Geometry: final body of the model. Coordinates: model frame, mm. A direction names the side the tool comes from. Give positions to 0.01 mm unless a question says otherwise; leave off trailing zeros. Order: outer loops, then holes, each group sorted by start corner. A loop starts at its lowest first (then second) coordinate and runs counter-clockwise, first axis right, second up. Notation, with made-up numbers: M -37.75,46.5 L -18.75,46.5 A22 cw -18.75,65.5 Z; hole C 48,59 d1. An arc over 180 degrees is marked long. Use CSV: the item, a comma, the result in double quotes.
```python
from build123d import *

# Parameters (mm, degrees)
SKETCH_2_R          = 1.65
SKETCH_2_R_2        = 6.3
EXTRUDE_1_DEPTH     = 5
SKETCH_4_W          = 4
SKETCH_4_H          = 55
EXTRUDE_3_DEPTH     = 54
CUT_EXTRUDE_1_DEPTH = 54


with BuildPart() as part:
    # 草图2 → 凸台-拉伸1 (new body)
    with BuildSketch(Plane.XY):
        Polygon((15.6, 35), (0, 35), (-15.6, 35), (-15.6, -20), (18.6, -20), (18.6, 35), align=None)
        with Locations((-9, -5)):
            Circle(SKETCH_2_R, mode=Mode.SUBTRACT)
        with Locations((0, -5)):
            Circle(SKETCH_2_R_2, mode=Mode.SUBTRACT)
        with Locations((9, -5)):
            Circle(SKETCH_2_R, mode=Mode.SUBTRACT)
    extrude(amount=EXTRUDE_1_DEPTH)

    # 草图4 → 凸台-拉伸3 (add)
    with BuildSketch(Plane.XY.offset(5)):
        with Locations((16.6, 7.5)):
            Rectangle(SKETCH_4_W, SKETCH_4_H)
    extrude(amount=EXTRUDE_3_DEPTH)

    # 草图6 → 切除-拉伸1 (cut)
    with BuildSketch(Plane(origin=(0, 0, 0), x_dir=(0, 0, -1), z_dir=(1, 0, 0))):
        Polygon((-59, 7.5), (-59, -20), (-5, -20), align=None)
        with BuildLine():
            ThreePointArc((-32.65, 20), (-31, 18.35), (-29.35, 20))
            Line((-29.35, 20), (-32.65, 20))
        make_face()
        with BuildLine():
            Line((-32.65, 20), (-29.35, 20))
            ThreePointArc((-29.35, 20), (-31, 21.65), (-32.65, 20))
        make_face()
        with BuildLine():
            ThreePointArc((-33.7, 20), (-40, 26.3), (-46.3, 20))
            Line((-46.3, 20), (-33.7, 20))
        make_face()
        with BuildLine():
            Line((-33.7, 20), (-46.3, 20))
            ThreePointArc((-46.3, 20), (-40, 13.7), (-33.7, 20))
        make_face()
        with BuildLine():
            ThreePointArc((-47.35, 20), (-49, 21.65), (-50.65, 20))
            Line((-50.65, 20), (-47.35, 20))
        make_face()
        with BuildLine():
            Line((-47.35, 20), (-50.65, 20))
            ThreePointArc((-50.65, 20), (-49, 18.35), (-47.35, 20))
        make_face()
    extrude(amount=CUT_EXTRUDE_1_DEPTH, mode=Mode.SUBTRACT)


solid = part.part
```
1. Pull-direction query (Z, two-part tool) for faces 1 (the face through (1, 8, 0)), 2 (the face through (16.572, 18.885, 47.784)), 3 (the face through (14.6, 13, 26)), 4 (the face through (16.572, 13.754, 39.18)); classes: +Z half, -Z half, draft (parallel to the pull), parting line (faces both ways), or undercut.
Answer:
face 1,"-Z half"
face 2,"undercut"
face 3,"draft"
face 4,"undercut"
2. Section D-D, the plane x = 11.5. Return the cut outline in (y, z), plus the area to 3 significant figures.
Answer:
outline,"M -20,0 L 35,0 L 35,5 L -20,5 Z"
area,"275 mm2"
3. Line query: line 1 (Y direction, x = -9, z = 2.15); line 2 (Y direction, x = 0, z = 3.8); line 3 (X direction, y = 11, z = 14.5). Output: solid intervals per line, ascending.
Answer:
line 1,"-20 to -6.65, -3.35 to 35"
line 2,"-20 to -11.3, 1.3 to 35"
line 3,"14.6 to 18.6"
4. Section B-B, the plane z = 43. Return the cut outline in (x, y), plus the area to 3 significant figures.
Answer:
outline,"M 14.6,-0.65 L 18.6,-0.65 L 18.6,14.46 L 14.6,14.46 Z; M 14.6,25.54 L 18.6,25.54 L 18.6,35 L 14.6,35 Z"
area,"98.3 mm2"
5. Section A-A, the plane x = 0. Return the cut outline in (y, z), plus the area to 3 significant figures.
Answer:
outline,"M -20,0 L -11.3,0 L -11.3,5 L -20,5 Z; M 1.3,0 L 35,0 L 35,5 L 1.3,5 Z"
area,"212 mm2"
6. Reachability of faces 5 (the face through (-1, 8, 5)), 6 (the face through (16.572, 21.115, 32.216)) from +Z, -Z, +X, -X, +Y, -Y: full face, straight path, thin tool, end or side. Return the list, or none.
Answer:
face 5,"+Z, -X, +Y, -Y"
face 6,"+X, -X"
7. Section C-C, the plane y = 31.5. Return the cut outline in (x, z), plus the area to 3 significant figures.
Answer:
outline,"M -15.6,0 L 18.6,0 L 18.6,59 L 14.6,59 L 14.6,5 L -15.6,5 Z"
area,"387 mm2"
8. Pin query (flat end, axial travel): pin 1 Ø3 at (y, z) = (20, 49) entering from +X; pin 2 Ø1 at (x, y) = (13.5, 14) entering from +Z; pin 3 Ø16 at (y, z) = (15.5, 26) entering from -X. Return the tip coordinate at first contact, or that it passes through.
Answer:
pin 1,"through"
pin 2,"z = 5"
pin 3,"x = 14.6"
